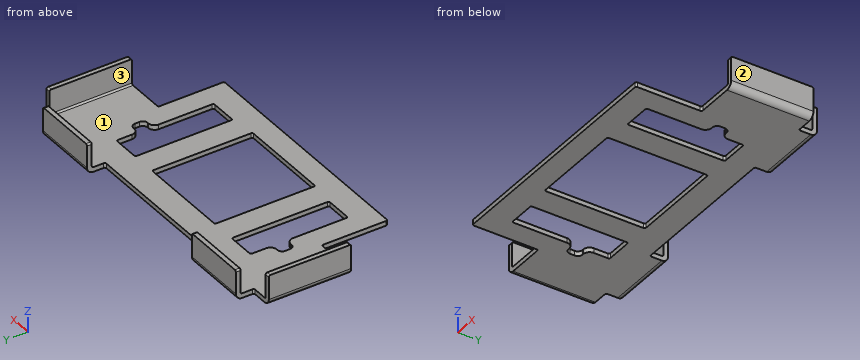
from build123d import *

# Parameters (mm, degrees)
SKETCH1_W           = 106
SKETCH1_H           = 26.2
BOSS_EXTRUDE1_DEPTH = 9.7
SKETCH2_W           = 103
SKETCH2_H           = 8.2
CUT_EXTRUDE1_DEPTH  = 27.2
SKETCH3_W           = 21
SKETCH3_H           = 1.5
BOSS_EXTRUDE2_DEPTH = 5.8
SKETCH4_W           = 21
SKETCH4_H           = 1.5
BOSS_EXTRUDE3_DEPTH = 8
SKETCH5_W           = 21
SKETCH5_H           = 1.5
BOSS_EXTRUDE4_DEPTH = 5.8
SKETCH6_W           = 21
SKETCH6_H           = 1.5
BOSS_EXTRUDE5_DEPTH = 8
SKETCH7_W           = 78
SKETCH7_H           = 1.5
BOSS_EXTRUDE6_DEPTH = 21
FILLET1_R           = 0.5
FILLET2_R           = 2
SKETCH8_W           = 30
SKETCH8_H           = 32
CUT_EXTRUDE2_DEPTH  = 1.5
FILLET4_R           = 2
FILLET5_R           = 1.5
FILLET6_R           = 0.5
FILLET7_R           = 0.5


with BuildPart() as part:
    # Sketch1 → Boss-Extrude1 (new body)
    with BuildSketch(Plane(origin=(0, 0, -42.5), x_dir=(-1, 0, 0), z_dir=(0, 0, -1))):
        with Locations((0, -2.9)):
            Rectangle(SKETCH1_W, SKETCH1_H)
    extrude(amount=-BOSS_EXTRUDE1_DEPTH)

    # Sketch2 → Cut-Extrude1 (cut, through all)
    with BuildSketch(Plane(origin=(0, 10.2, 0), x_dir=(-1, 0, 0), z_dir=(0, 1, 0))):
        with Locations((0, -36.9)):
            Rectangle(SKETCH2_W, SKETCH2_H)
    extrude(amount=-CUT_EXTRUDE1_DEPTH, mode=Mode.SUBTRACT)

    # Sketch3 → Boss-Extrude2 (add)
    with BuildSketch(Plane(origin=(0, 10.2, 0), x_dir=(-1, 0, 0), z_dir=(0, 1, 0))):
        with Locations((35.5, -41.75)):
            Rectangle(SKETCH3_W, SKETCH3_H)
    extrude(amount=BOSS_EXTRUDE2_DEPTH)

    # Sketch4 → Boss-Extrude3 (add)
    with BuildSketch(Plane.XY.offset(-41)):
        with Locations((-35.5, 15.25)):
            Rectangle(SKETCH4_W, SKETCH4_H)
    extrude(amount=BOSS_EXTRUDE3_DEPTH)

    # Sketch5 → Boss-Extrude4 (add)
    with BuildSketch(Plane(origin=(0, 10.2, 0), x_dir=(-1, 0, 0), z_dir=(0, 1, 0))):
        with Locations((-35.5, -41.75)):
            Rectangle(SKETCH5_W, SKETCH5_H)
    extrude(amount=BOSS_EXTRUDE4_DEPTH)

    # Sketch6 → Boss-Extrude5 (add)
    with BuildSketch(Plane.XY.offset(-41)):
        with Locations((35.5, 15.25)):
            Rectangle(SKETCH6_W, SKETCH6_H)
    extrude(amount=BOSS_EXTRUDE5_DEPTH)

    # Sketch7 → Boss-Extrude6 (add)
    with BuildSketch(Plane.XZ.offset(16)):
        with Locations((0, -41.75)):
            Rectangle(SKETCH7_W, SKETCH7_H)
    extrude(amount=BOSS_EXTRUDE6_DEPTH)

    # Fillet1
    fillet1_edges = [part.edges().sort_by_distance(p)[0] for p in [
        (-51.5, -2.9, -41),
        (51.5, -2.9, -41),
        (-35.5, 14.5, -41),
        (35.5, 14.5, -41),
    ]]
    fillet(fillet1_edges, radius=FILLET1_R)

    # Fillet2
    fillet2_edges = [part.edges().sort_by_distance(p)[0] for p in [
        (-35.5, 16, -42.5),
        (53, -2.9, -42.5),
        (-53, -2.9, -42.5),
        (35.5, 16, -42.5),
    ]]
    fillet(fillet2_edges, radius=FILLET2_R)

    # Sketch8 → Cut-Extrude2 (cut)
    with BuildSketch(Plane(origin=(0, 0, -42.5), x_dir=(-1, 0, 0), z_dir=(0, 0, -1))):
        with Locations((0, -14)):
            Rectangle(SKETCH8_W, SKETCH8_H)
        Polygon((-23, 2), (-32, 2), (-32, -5), (-35.831359268, -5), (-35.831359268, -9.5), (-32, -9.5), (-32, -29), (-23, -29), align=None)
        Polygon((32, -29), (23, -29), (23, 2), (32, 2), (32, -5), (35.831359268, -5), (35.831359268, -9.5), (32, -9.5), align=None)
    extrude(amount=-CUT_EXTRUDE2_DEPTH, mode=Mode.SUBTRACT)

    # Fillet4
    fillet4_edges = [part.edges().sort_by_distance(p)[0] for p in [
        (32, -9.5, -41.75),
        (32, -5, -41.75),
        (-32, -9.5, -41.75),
        (-32, -5, -41.75),
    ]]
    fillet(fillet4_edges, radius=FILLET4_R)

    # Fillet5
    fillet5_edges = [part.edges().sort_by_distance(p)[0] for p in [
        (35.831359268, -9.5, -41.75),
        (35.831359268, -5, -41.75),
        (-35.831359268, -5, -41.75),
        (-35.831359268, -9.5, -41.75),
    ]]
    fillet(fillet5_edges, radius=FILLET5_R)

    # Fillet6
    fillet6_edges = [part.edges().sort_by_distance(p)[0] for p in [
        (15, -30, -41.75),
        (15, 2, -41.75),
        (-15, 2, -41.75),
        (-15, -30, -41.75),
        (23, 2, -41.75),
        (23, -29, -41.75),
        (32, -29, -41.75),
        (32, 2, -41.75),
        (-32, -29, -41.75),
        (-23, -29, -41.75),
        (-23, 2, -41.75),
        (-32, 2, -41.75),
    ]]
    fillet(fillet6_edges, radius=FILLET6_R)

    # Fillet7
    fillet7_edges = [part.edges().sort_by_distance(p)[0] for p in [
        (52.25, -16, -32.8),
        (-52.25, -16, -32.8),
        (52.25, 10.2, -32.8),
        (-25, 10.2, -41.75),
        (-46, 10.2, -41.75),
        (-46, 15.25, -33),
        (-25, 15.25, -33),
        (46, 10.2, -41.75),
        (25, 10.2, -41.75),
        (-52.25, 10.2, -32.8),
        (46, 15.25, -33),
        (25, 15.25, -33),
        (-39, -16, -41.75),
        (39, -16, -41.75),
        (-39, -37, -41.75),
        (39, -37, -41.75),
    ]]
    fillet(fillet7_edges, radius=FILLET7_R)


solid = part.part
Verification items for the finished model (mm, model axes). Face numbers are marked on the shaded views. A direction names the side the tool comes from. Coordinates: 2 decimals unless noted, no trailing zeros. Loops run counter-clockwise (first coordinate to the right, second up) from the corner with the lowest first, then second, coordinate; pieces in that order, holes last. Notation, with made-up numbers: (20, 70) -> (56, 70) arc R10 ccw to (56, 75) -> close; hole circle Ø11 at (84.5, 76). An arc over 180 degrees is marked (long way). Answer as CSV lines item,"result".
1) Cross-section at A-A, the plane x = 30. Record the cut outline in (y, z).
Found:
outline,"(-37, -42.5) -> (-29, -42.5) -> (-29, -41) -> (-37, -41) -> close; (2, -42.5) -> (14, -42.5) arc R2 ccw to (16, -40.5) -> (16, -33) -> (14.5, -33) -> (14.5, -40.5) arc R0.5 cw to (14, -41) -> (2, -41) -> close"
2) Cross-section at B-B, the plane y = -14. Record the cut outline in (x, z).
Found:
outline,"(-53, -40.5) arc R2 ccw to (-51, -42.5) -> (-32, -42.5) -> (-32, -41) -> (-51, -41) arc R0.5 cw to (-51.5, -40.5) -> (-51.5, -32.8) -> (-53, -32.8) -> close; (-23, -42.5) -> (-15, -42.5) -> (-15, -41) -> (-23, -41) -> close; (15, -42.5) -> (23, -42.5) -> (23, -41) -> (15, -41) -> close; (32, -42.5) -> (51, -42.5) arc R2 ccw to (53, -40.5) -> (53, -32.8) -> (51.5, -32.8) -> (51.5, -40.5) arc R0.5 cw to (51, -41) -> (32, -41) -> close"
3) Cross-section at D-D, the plane x = -6.5. Record the cut outline in (y, z).
Found:
outline,"(-37, -42.5) -> (-30, -42.5) -> (-30, -41) -> (-37, -41) -> close; (2, -42.5) -> (10.2, -42.5) -> (10.2, -41) -> (2, -41) -> close"
4) Depth check by flat-ended pin: pin 1 (1.6 mm diameter, centred on x = 9.5, z = -41.5, fed in from +Y); pin 2 (0.8 mm diameter, centred on x = 27, z = -41.5, fed in from +Y); pin 3 (4 mm diameter, centred on y = 14, z = -40, fed in from -X). Enter the tip coordinate at first touch or a pass-through.
Found:
pin 1,"stops at y = 10.2"
pin 2,"stops at y = 15.91"
pin 3,"stops at x = -46"
5) Thickness scan on L1, parallel to X at y = 6.5, z = -33.75; L2, parallel to Y at x = 27.5, z = -38.75; L3, parallel to Z at x = 46.5, y = 4.5. Record the ranges inside material, lowest first. Write a range as from..to.
Found:
L1,"x = -53..-51.5, 51.5..53"
L2,"y = 14.5..16"
L3,"z = -42.5..-41"
6) Tool access check on the marked faces 1, 2 and 3. Record the directions out of +Z, -Z, +X, -X, +Y, -Y that give a thin tool (end or side, any length) a straight path to the whole face; none if there is none.
Found:
face 1,"+Z, -Y"
face 2,"+Z, -Z, +X, +Y, -Y"
face 3,"+Z, +Y, -Y"
7) Cross-section at C-C, the plane z = -38.75. Record the cut outline in (x, y), then the cut area to 3 significant figures.
Found:
outline,"(-53, -16) -> (-51.5, -16) -> (-51.5, 10.2) -> (-53, 10.2) -> close; (-46, 14.5) -> (-25, 14.5) -> (-25, 16) -> (-46, 16) -> close; (25, 14.5) -> (46, 14.5) -> (46, 16) -> (25, 16) -> close; (51.5, -16) -> (53, -16) -> (53, 10.2) -> (51.5, 10.2) -> close"
area,"142 mm2"
